Drawing for the job (mm, zero at the part's lowest x, y, z). A direction names the side the tool comes from. Give positions to 0.01 mm unless a question says otherwise; leave off trailing zeros. Order: outer loops, then holes, each group sorted by start corner. A loop starts at its lowest first (then second) coordinate and runs counter-clockwise, first axis right, second up. Notation, with made-up numbers: (13.25, 17) - (45.25, 17) arc R23 ccw to (45.25, 54) - close; hole circle Ø3 at (56.25, 12). An arc over 180 degrees is marked (long way). Use CSV: the item, a comma, the result in double quotes. Start each with the question number.
(1) Pull direction Y, two halves, no side cores. Call the marked faces 3, 4 and 5: +Y half, -Y half, draft (parallel to the pull), parting line (faces both ways), or undercut.
(2) Tool access for the marked faces 1 and 2: list every direction of +Z, -Z, +X, -X, +Y, -Y with a clear straight run to the whole face (end or side of a thin tool).
(3) Probe L1, parallel to Y at x = 52, z = 30.5; L2, parallel to Y at x = 5.5, z = 42.5; L3, parallel to Y at x = 48.5, z = 8.5. List the from-to ranges inside material, lowest first.
(4) Band-saw the part on B-B, the plane x = 48.5. Give the cut face in (y, z).
(5) Band-saw the part on A-A, the plane z = 33.5. Give the cut face in (x, y), then the cut area to 3 significant figures.
(6) Drop a flat-ended pin along its axis: pin 1 Ø7 at (x, z) = (48, 35) entering from +Y. Give the stop position or say it passes through.
(7) Band-saw the part on C-C, the plane y = 337.5. Give the cut face in (x, z), then the cut area to 3 significant figures.
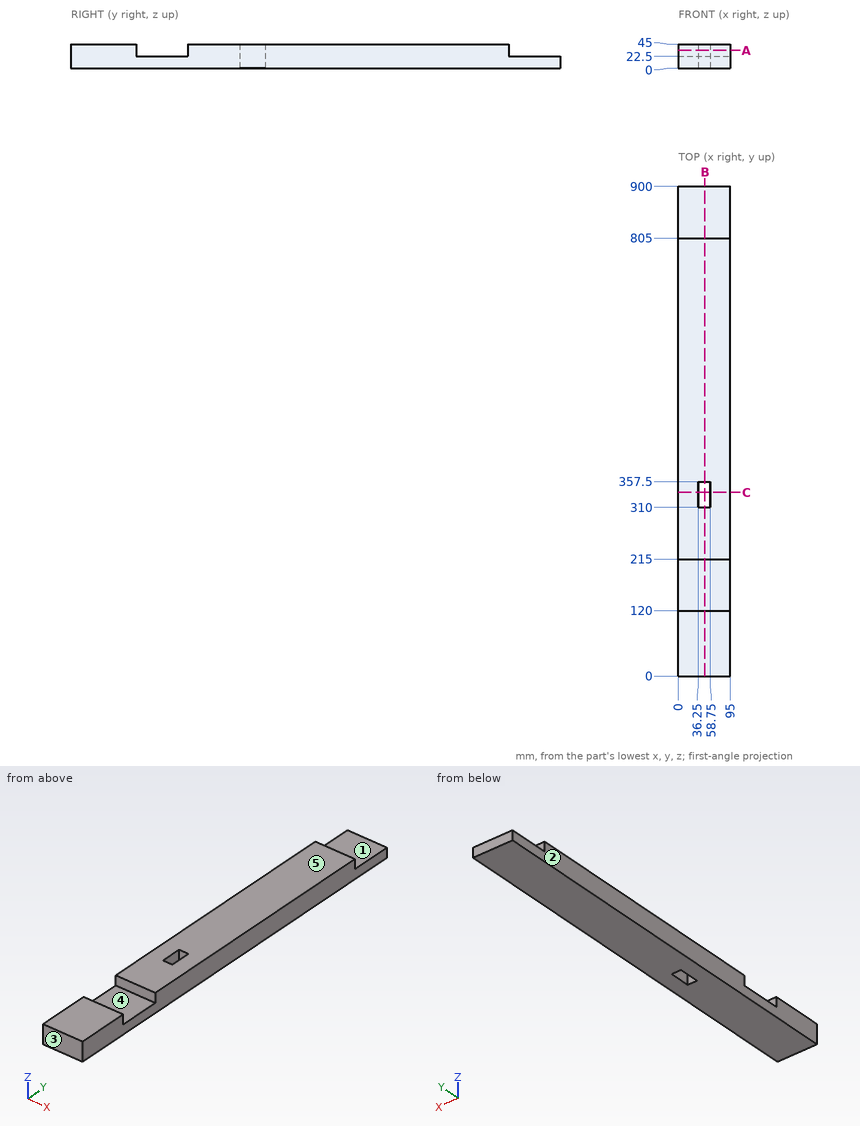
Answer block:
1,face 3,"-Y half"
1,face 4,"undercut"
1,face 5,"draft"
2,face 1,"+Z, +X, -X, +Y"
2,face 2,"+Z, -Z, -X, +Y, -Y"
3,L1,"y = 0 to 120, 215 to 310, 357.5 to 805"
3,L2,"y = 0 to 120, 215 to 805"
3,L3,"y = 0 to 310, 357.5 to 900"
4,outline,"(0, 0) - (310, 0) - (310, 45) - (215, 45) - (215, 22.5) - (120, 22.5) - (120, 45) - (0, 45) - close; (357.5, 0) - (900, 0) - (900, 22.5) - (805, 22.5) - (805, 45) - (357.5, 45) - close"
5,outline,"(0, 0) - (95, 0) - (95, 120) - (0, 120) - close; (0, 215) - (95, 215) - (95, 805) - (0, 805) - close; hole (36.25, 310) - (58.75, 310) - (58.75, 357.5) - (36.25, 357.5) - close"
5,area,"66,400 mm2"
6,pin 1,"stops at y = 805"
7,outline,"(0, 0) - (36.25, 0) - (36.25, 45) - (0, 45) - close; (58.75, 0) - (95, 0) - (95, 45) - (58.75, 45) - close"
7,area,"3,260 mm2"
